from build123d import *

# Parameters (mm, degrees)
SKETCH2_R           = 6.96865511
BOSS_EXTRUDE1_DEPTH = 25
SKETCH3_W           = 38.455930717
SKETCH3_H           = 55.217032342
CUT_EXTRUDE1_DEPTH  = 109.000086758
FILLET1_RADIUS      = 25
FILLET1_LENGTH      = 12.285129205
FILLET2_R           = 10
FILLET3_R           = 10
FILLET4_R           = 10
FILLET5_R           = 10


with BuildPart() as part:
    # Sketch2 → Boss-Extrude1 (new, symmetric)
    with BuildSketch(Plane.XY):
        with BuildLine():
            Line((0, 0), (50.197302129, 0))
            ThreePointArc((50.197302129, 0), (61.607367951, 18.906462701), (80.513830652, 30.316528523))
            Line((80.513830652, 30.316528523), (80.513830652, 67.502161547))
            Line((80.513830652, 67.502161547), (48.421245481, 67.502161547))
            Line((48.421245481, 67.502161547), (27.021342994, 12.285129205))
            Line((27.021342994, 12.285129205), (0, 12.285129205))
            Line((0, 12.285129205), (0, 0))
        make_face()
        with Locations((62.192399066, 49.399617147)):
            Circle(SKETCH2_R, mode=Mode.SUBTRACT)
    extrude(amount=BOSS_EXTRUDE1_DEPTH, both=True)

    # Sketch3 → Cut-Extrude1 (cut, through all)
    with BuildSketch(Plane(origin=(0, 0, 0), x_dir=(0, 0, -1), z_dir=(1, 0, 0))):
        with Locations((-0.137670396, 39.893645376)):
            Rectangle(SKETCH3_W, SKETCH3_H)
    extrude(amount=CUT_EXTRUDE1_DEPTH, mode=Mode.SUBTRACT)

    # Fillet1: full round fillet: the end face becomes a half cylinder, R = half its width
    fillet1_face = Plane((0, 6.142564603, 0), x_dir=(0, -1, 0), z_dir=(-1, 0, 0))  # on the end face: x along it, z out of the body
    fillet1_slab = fillet1_face.offset(-FILLET1_RADIUS / 2) * Box(FILLET1_LENGTH, 2 * FILLET1_RADIUS, FILLET1_RADIUS, mode=Mode.PRIVATE)  # the body's end, R deep
    fillet1_round = Plane((25, 6.142564603, 0), x_dir=(-1, 0, 0), z_dir=(0, -1, 0)) * Cylinder(FILLET1_RADIUS, FILLET1_LENGTH, mode=Mode.PRIVATE)  # its axis R under the face
    add(fillet1_slab - fillet1_round, mode=Mode.SUBTRACT)

    # Fillet2
    fillet2_edges = [part.edges().sort_by_distance(p)[0] for p in [
        (48.421245481, 67.502161547, -22.045147481),
    ]]
    fillet(fillet2_edges, radius=FILLET2_R)

    # Fillet3
    fillet3_edges = [part.edges().sort_by_distance(p)[0] for p in [
        (80.513830652, 67.502161547, -22.045147481),
    ]]
    fillet(fillet3_edges, radius=FILLET3_R)

    # Fillet4
    fillet4_edges = [part.edges().sort_by_distance(p)[0] for p in [
        (48.421245481, 67.502161547, 22.182817878),
    ]]
    fillet(fillet4_edges, radius=FILLET4_R)

    # Fillet5
    fillet5_edges = [part.edges().sort_by_distance(p)[0] for p in [
        (80.513830652, 67.502161547, 22.182817878),
    ]]
    fillet(fillet5_edges, radius=FILLET5_R)

    # Sketch6 → 3/4 NPT Tapped Hole1 (revolve, cut)
    with BuildSketch(Plane(origin=(24.396705522, 12.285129205, -1.643830205), x_dir=(0, 0, 1), z_dir=(1, 0, 0))):
        Polygon((0, 0), (0, 12.285129205), (11.5062, 12.285129205), (11.5062, 14.05), (12.137858885, 14.05), (12.5585347, 0), align=None)
    revolve(axis=Axis((24.396705522, 18.635129205, -1.643830205), (0, -1, 0)), mode=Mode.SUBTRACT)


solid = part.part
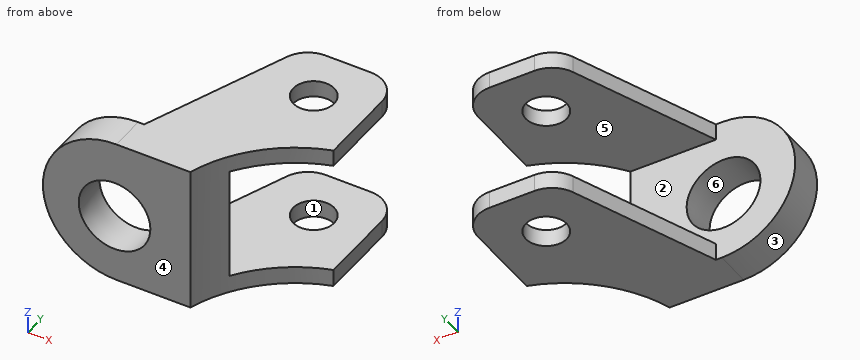
Geometry: final body of the model. Coordinates: model frame, mm. Face numbers are marked on the shaded views. A direction names the side the tool comes from. Give positions to 0.01 mm unless a question says otherwise; leave off trailing zeros. Loops run counter-clockwise (first coordinate to the right, second up) from the corner with the lowest first, then second, coordinate; pieces in that order, holes last. Notation, with made-up numbers: M 63.5,-3 L 71.5,-3 A12 ccw 71.5,15 Z; hole C -0.75,-12 d7. An arc over 180 degrees is marked long. Put each result on its own line as item: value. Start each with the question number.
1) Ray query, line 1 along Z through (x, y) = (56, 26.5); line 2 along Y through (x, z) = (33, -12); line 3 along X through (y, z) = (46, 21.5). Return the intervals inside material, ascending.
2) Cut plane D-D (y = 29). Output: boundary loops of the cut face in (x, z).
3) Cut plane B-B (z = -21.5). Output: boundary loops of the cut face in (x, y), then the cut area to 3 significant figures.
4) Cut plane C-C (x = 45). Output: boundary loops of the cut face in (y, z).
5) Contact query for flat-ended pins moving along their axis: pin 1 (8 mm diameter, centred on x = 59.5, z = 1.5, fed in from +Y); pin 2 (5 mm diameter, centred on y = 13.5, z = -1, fed in from +X). Output: stop coordinate, or through.
6) Pull-direction query (Z, two-part tool) for the marked faces 1, 2 and 3; classes: pulls with the +Z half, pulls with the -Z half, needs draft (parallel to the pull), parting line crosses it, or undercut.
7) Access query for the marked faces 4, 5 and 6. Directions: +Z, -Z, +X, -X, +Y, -Y. A direction counts if a zero-diameter tool reaches every point of the face in a straight line with its end or side. Return the directions, or none.
8) Cut plane A-A (y = 39.5). Output: boundary loops of the cut face in (x, z), then the cut area to 3 significant figures.
Verdict:
1. line 1: -25 to -19.09, 19.37 to 25
1. line 2: 0 to 12.29
1. line 3: 40.09 to 56.11, 68.28 to 80.51
2. outline: M 33.5,-25 L 76.83,-25 L 76.83,-19.09 L 33.5,-19.09 Z; M 33.5,19.37 L 76.83,19.37 L 76.83,25 L 33.5,25 Z
3. outline: M 12.24,0 L 50.2,0 A46 cw 80.51,30.32 L 80.51,57.5 A10 ccw 70.51,67.5 L 55.27,67.5 A10 ccw 45.95,61.12 L 27.02,12.29 L 12.24,12.29 Z; hole C 62.19,49.4 d13.94
3. area: 2,410 mm2
4. outline: M 0,-25 L 58.67,-25 L 58.67,-19.09 L 12.29,-19.09 L 12.29,19.37 L 58.67,19.37 L 58.67,25 L 0,25 Z
5. pin 1: y = 12.29
5. pin 2: x = 56.12
6. face 1: needs draft
6. face 2: undercut
6. face 3: parting line crosses it
7. face 4: +Z, -Z, +X, -X, -Y
7. face 5: +X, -X, +Y
7. face 6: +Y
8. outline: M 37.57,-25 L 80.51,-25 L 80.51,-19.09 L 37.57,-19.09 Z; M 37.57,19.37 L 80.51,19.37 L 80.51,25 L 37.57,25 Z
8. area: 496 mm2
